Can you work these out from the model? Positions are in its coordinate system, mm. Round coordinates to 2 decimals unless told otherwise and drop trailing zeros. Order: outer loops, then holes, each group sorted by start corner. A loop starts at its lowest first (then second) coordinate and runs counter-clockwise, first axis right, second up. Notation, with made-up numbers: M 0.5,-9 L 16.5,-9 A20 ccw 16.5,-4 Z; hole C 2,-1 d2. An arc over 180 degrees is marked long. One line per question, with ' | ' between items.
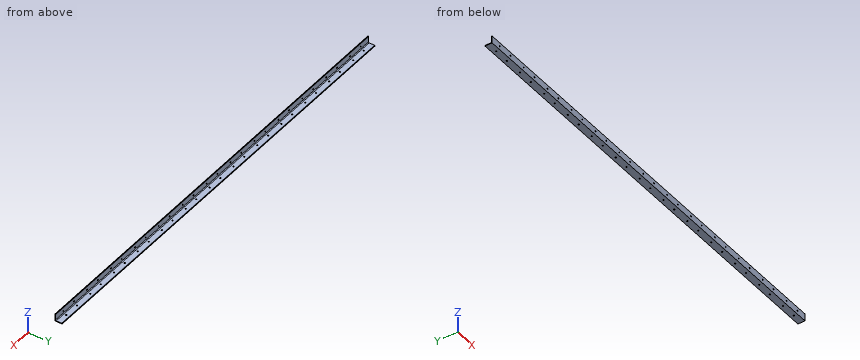
```python
from build123d import *

# Parameters (mm, degrees)
F1_DEPTH      = 1090
F1_DEPTH_BACK = 1090
F2_R          = 3
F3_DEPTH      = 25
F4_R          = 3
F5_DEPTH      = 25


with BuildPart() as f1:
    # F0 (on Right) → F1 (new body, two sides)
    with BuildSketch(Plane.YZ) as f1_sk:
        with BuildLine():
            Line((0, 35), (0, 0))
            Line((0, 0), (35, 0))
            Line((35, 0), (35, 1))
            ThreePointArc((35, 1), (34.414214, 2.414214), (33, 3))
            Line((33, 3), (6.5, 3))
            ThreePointArc((6.5, 3), (4.025126, 4.025126), (3, 6.5))
            Line((3, 6.5), (3, 33))
            ThreePointArc((3, 33), (2.414214, 34.414214), (1, 35))
            Line((1, 35), (0, 35))
        make_face()
    extrude(amount=F1_DEPTH)
    extrude(f1_sk.sketch, amount=-F1_DEPTH_BACK)

    # F2 (on face) → F3 (cut)
    with BuildSketch(Plane.XZ):
        with Locations((1128, 17.5)):
            Circle(F2_R)
        with Locations((1203, 17.5)):
            Circle(F2_R)
        with Locations((1294.5, 17.5)):
            Circle(F2_R)
        with Locations((1369.5, 17.5)):
            Circle(F2_R)
        with Locations((1461, 17.5)):
            Circle(F2_R)
        with Locations((1536, 17.5)):
            Circle(F2_R)
        with Locations((1627.5, 17.5)):
            Circle(F2_R)
        with Locations((1702.5, 17.5)):
            Circle(F2_R)
        with Locations((1794, 17.5)):
            Circle(F2_R)
        with Locations((1869, 17.5)):
            Circle(F2_R)
        with Locations((1960.5, 17.5)):
            Circle(F2_R)
        with Locations((2035.5, 17.5)):
            Circle(F2_R)
        with Locations((2127, 17.5)):
            Circle(F2_R)
        with Locations((2202, 17.5)):
            Circle(F2_R)
        with Locations((-961.5, 17.5)):
            Circle(F2_R)
        with Locations((-870, 17.5)):
            Circle(F2_R)
        with Locations((-795, 17.5)):
            Circle(F2_R)
        with Locations((-703.5, 17.5)):
            Circle(F2_R)
        with Locations((-628.5, 17.5)):
            Circle(F2_R)
        with Locations((-537, 17.5)):
            Circle(F2_R)
        with Locations((-462, 17.5)):
            Circle(F2_R)
        with Locations((-370.5, 17.5)):
            Circle(F2_R)
        with Locations((-295.5, 17.5)):
            Circle(F2_R)
        with Locations((-204, 17.5)):
            Circle(F2_R)
        with Locations((-129, 17.5)):
            Circle(F2_R)
        with Locations((-37.5, 17.5)):
            Circle(F2_R)
        with Locations((37.5, 17.5)):
            Circle(F2_R)
        with Locations((129, 17.5)):
            Circle(F2_R)
        with Locations((204, 17.5)):
            Circle(F2_R)
        with Locations((295.5, 17.5)):
            Circle(F2_R)
        with Locations((370.5, 17.5)):
            Circle(F2_R)
        with Locations((462, 17.5)):
            Circle(F2_R)
        with Locations((537, 17.5)):
            Circle(F2_R)
        with Locations((628.5, 17.5)):
            Circle(F2_R)
        with Locations((703.5, 17.5)):
            Circle(F2_R)
        with Locations((795, 17.5)):
            Circle(F2_R)
        with Locations((870, 17.5)):
            Circle(F2_R)
        with Locations((961.5, 17.5)):
            Circle(F2_R)
        with Locations((1036.5, 17.5)):
            Circle(F2_R)
        with Locations((-1036.5, 17.5)):
            Circle(F2_R)
    extrude(amount=-F3_DEPTH, mode=Mode.SUBTRACT)

    # F4 (on face) → F5 (cut)
    with BuildSketch(Plane(origin=(0, 0, 0), x_dir=(1, 0, 0), z_dir=(0, 0, -1))):
        with Locations((-1036.5, -17.5)):
            Circle(F4_R)
        with Locations((-961.5, -17.5)):
            Circle(F4_R)
        with Locations((-870, -17.5)):
            Circle(F4_R)
        with Locations((-795, -17.5)):
            Circle(F4_R)
        with Locations((-703.5, -17.5)):
            Circle(F4_R)
        with Locations((-628.5, -17.5)):
            Circle(F4_R)
        with Locations((-537, -17.5)):
            Circle(F4_R)
        with Locations((-462, -17.5)):
            Circle(F4_R)
        with Locations((-370.5, -17.5)):
            Circle(F4_R)
        with Locations((-295.5, -17.5)):
            Circle(F4_R)
        with Locations((-204, -17.5)):
            Circle(F4_R)
        with Locations((-129, -17.5)):
            Circle(F4_R)
        with Locations((-37.5, -17.5)):
            Circle(F4_R)
        with Locations((37.5, -17.5)):
            Circle(F4_R)
        with Locations((129, -17.5)):
            Circle(F4_R)
        with Locations((204, -17.5)):
            Circle(F4_R)
        with Locations((295.5, -17.5)):
            Circle(F4_R)
        with Locations((370.5, -17.5)):
            Circle(F4_R)
        with Locations((462, -17.5)):
            Circle(F4_R)
        with Locations((537, -17.5)):
            Circle(F4_R)
        with Locations((628.5, -17.5)):
            Circle(F4_R)
        with Locations((703.5, -17.5)):
            Circle(F4_R)
        with Locations((795, -17.5)):
            Circle(F4_R)
        with Locations((870, -17.5)):
            Circle(F4_R)
        with Locations((961.5, -17.5)):
            Circle(F4_R)
        with Locations((1036.5, -17.5)):
            Circle(F4_R)
        with Locations((1128, -17.5)):
            Circle(F4_R)
        with Locations((1203, -17.5)):
            Circle(F4_R)
        with Locations((1294.5, -17.5)):
            Circle(F4_R)
        with Locations((1369.5, -17.5)):
            Circle(F4_R)
        with Locations((1461, -17.5)):
            Circle(F4_R)
        with Locations((1536, -17.5)):
            Circle(F4_R)
        with Locations((1627.5, -17.5)):
            Circle(F4_R)
        with Locations((1702.5, -17.5)):
            Circle(F4_R)
        with Locations((1794, -17.5)):
            Circle(F4_R)
        with Locations((1869, -17.5)):
            Circle(F4_R)
        with Locations((1960.5, -17.5)):
            Circle(F4_R)
        with Locations((2035.5, -17.5)):
            Circle(F4_R)
        with Locations((2127, -17.5)):
            Circle(F4_R)
        with Locations((2202, -17.5)):
            Circle(F4_R)
    extrude(amount=-F5_DEPTH, mode=Mode.SUBTRACT)


solid = f1.part
```
(1) Will these pins go through, and if not, where does the flat tip stop? pin 1 Ø7 at (x, z) = (-703.5, 17.5) entering from +Y; pin 2 Ø5.5 at (x, z) = (703.5, 17.5) entering from +Y.
Final values:
pin 1: y = 3 | pin 2: through
(2) If we section it at A-A on x = 906.5: Please give me the cut outline in (y, z), plus the area to 3 significant figures.
Final values:
outline: M 0,0 L 35,0 L 35,1 A2 ccw 33,3 L 6.5,3 A3.5 cw 3,6.5 L 3,33 A2 ccw 1,35 L 0,35 Z | area: 202 mm^2
(3) Please list where these lines run through material, in increasing order: probe 1 along Y at (x, z) = (-537, 2); probe 2 along Z at (x, y) = (795, 1); probe 3 along Y at (x, z) = (742.5, 16). Write a range as [from, to].
Final values:
probe 1: [0, 14.5], [20.5, 34.73] | probe 2: [0, 14.5], [20.5, 35] | probe 3: [0, 3]
